The model under review builds one solid part; all positions refer to its coordinate system, in mm. Face numbers are marked on the shaded views. A direction names the side the tool comes from. Round coordinates to 2 decimals unless told otherwise and drop trailing zeros. Order: outer loops, then holes, each group sorted by start corner. A loop starts at its lowest first (then second) coordinate and runs counter-clockwise, first axis right, second up. Notation, with made-up numbers: M 45,35.25 L 71,35.25 A22 ccw 71,41.25 Z; hole C -2,-25.5 d4. An arc over 180 degrees is marked long. One line per item, written item: value. Start each with the question number.
Autodesk Inventor part; units mm, degrees
ref_plane "YZ Plane" through (0, 0, 0) normal (1, 0, 0) x (0, 1, 0)
ref_plane "XZ Plane" through (0, 0, 0) normal (0, 1, 0) x (-1, 0, 0)
ref_plane "XY Plane" through (0, 0, 0) normal (0, 0, 1) x (1, 0, 0)
sketch "Sketch1" plane through (0, 0, 0) normal (0, 0, 1) x (1, 0, 0)
  circle A0 centre (0, 0) radius 28
  circle A1 centre (0, 0) radius 14
  circle A2 centre (0, 0) radius 19
  line L0 (0, 0) -> (-24.2487, 14)
  line L1 (0, 0) -> (24.2487, 14)
  line L2 (0, 0) -> (6.8345, 0)
  line L3 (0, 0) -> (24.2487, -14)
  line L4 (0, 0) -> (-24.2487, -14)
  point P0 (-16.4545, 9.5)
  point P1 (16.4545, 9.5)
  point P2 (-16.4545, -9.5)
  point P3 (16.4545, -9.5)
  dimension "d0" = 56
  dimension "d1" = 28
  dimension "d2" = 5
  dimension "d3" = 120
  dimension "d4" = 30
  dimension "d8" = 120
  dimension "d9" = 60
extrude "Extrusion1" add sketch "Sketch1" along normal blind 10 contours L1 A2 L0 A0 | L1 A1 L0 A2 | A2 L3 A1 L1 | A2 L4 A1 L3 | L0 A1 L4 A2
fillet "Fillet1" radius 1 2 edges at (-14, 0, 0) (-14, 0, 10)
extrude "Extrusion2" add sketch "Sketch1" along normal blind 10 contours A0 L4 A2 L3
properties part number "soporte bomba"
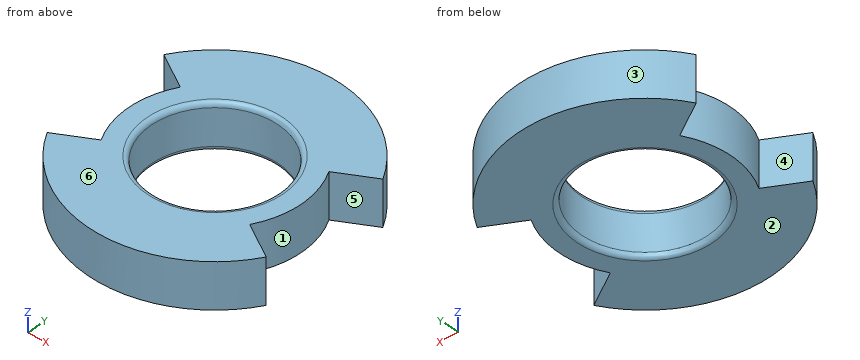
Item 1: Clearance check with flat-ended pins moving along their axes: P1, Ø2, axis at x = 2.5, z = 8, coming from the -Y side; P2, Ø1.5, axis at y = -4, z = 5.5, coming from the -X side; P3, Ø5, axis at y = -3.5, z = 4, coming from the +X side. State where each tip first meets the part, or that it passes through.
Item 2: Consider section B-B, the plane x = 0. Give the boundary of the cut face in (y, z).
Item 3: Machinability: for the marked faces 4, 5 and 6, which of the approach directions +Z, -Z, +X, -X, +Y, -Y give a long, thin tool a straight path to every point of the face, cutting with its end or side? Answer none if there is none.
Item 4: Consider section A-A, the plane y = 0. Give the boundary of the cut face in (x, z), then the cut area to 3 significant figures.
Item 5: Wall thickness on L1, parallel to X at y = 0, z = 2.5; L2, parallel to Y at x = -0.5, z = 5; L3, parallel to Y at x = -17.5, z = 8.75: over which ranges is each line inside the solid? List them lowest first.
Item 6: Consider section C-C, the plane z = 2. Give the boundary of the cut face in (x, y).
Item 7: The part is to be moulded in two halves that separate along Y. For the marked faces 1, 2 and 3, say which applies: pulls with the +Y half, pulls with the -Y half, needs draft (parallel to the pull), parting line crosses it, or undercut.
Item 8: Consider section D-D, the plane y = -24. Give the boundary of the cut face in (x, z), then the cut area to 3 significant figures.
Computed:
1. P1: stops at y = -27.96
1. P2: stops at x = -18.72
1. P3: stops at x = 18.97
2. outline: M -28,0 L -15,0 A1 ccw -14,1 L -14,9 A1 ccw -15,10 L -28,10 Z; M 14,1 A1 ccw 15,0 L 28,0 L 28,10 L 15,10 A1 ccw 14,9 Z
3. face 4: +Z, -Z, -X
3. face 5: +Z, -Z, +X
3. face 6: +Z, +X, -X, +Y, -Y
4. outline: M -19,0 L -15,0 A1 ccw -14,1 L -14,9 A1 ccw -15,10 L -19,10 Z; M 14,1 A1 ccw 15,0 L 19,0 L 19,10 L 15,10 A1 ccw 14,9 Z
4. area: 99.1 mm^2
5. L1: x = -19 to -14, 14 to 19
5. L2: y = -28 to -13.99, 13.99 to 28
5. L3: y = -21.86 to -10.1, -7.4 to 7.4, 10.1 to 21.86
6. outline: M -24.25,-14 A28 ccw 24.25,-14 L 16.45,-9.5 A19 ccw 16.45,9.5 L 24.25,14 A28 ccw -24.25,14 L -16.45,9.5 A19 ccw -16.45,-9.5 Z; hole C 0,0 d28
7. face 1: undercut
7. face 2: needs draft
7. face 3: pulls with the +Y half
8. outline: M -14.42,0 L 14.42,0 L 14.42,10 L -14.42,10 Z
8. area: 288 mm^2
